Geometry check sheet. Reference: the model listing, model coordinates, mm. Face numbers are marked on the shaded views. A direction names the side the tool comes from. Round coordinates to 2 decimals unless told otherwise and drop trailing zeros. Write each loop counter-clockwise with the first axis right and the second up, starting at its lowest first coordinate (ties: lowest second). Pieces come first, ordered by that corner, then holes. Notation, with made-up numbers: M 68.25,69 L 91.25,69 A30 ccw 91.25,101 Z; hole C 55,23.25 d2. An arc over 180 degrees is marked long. Use a Markdown table: item, result.
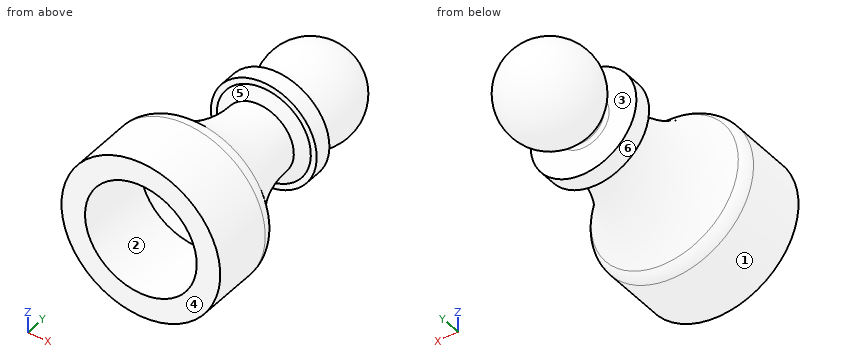
```python
from build123d import *

# Parameters (mm, degrees)
CHAMFER1_SIZE = 2
FILLET1_R     = 3
FILLET2_R     = 0.5


with BuildPart() as part:
    # Sketch1 → Revolve1 (revolve)
    with BuildSketch(Plane.XY, mode=Mode.PRIVATE) as revolve1_sk:
        with BuildLine():
            Line((9.5, 13.045692134), (9.5, 0))
            Line((9.5, 0), (13.5, 0))
            Line((13.5, 0), (13.5, 12))
            ThreePointArc((13.5, 12), (7.655959241, 19.576158489), (6, 29))
            Line((6, 29), (9, 29))
            Line((9, 29), (9, 32))
            Line((9, 32), (3.872983346, 32))
            Line((3.872983346, 32), (3.872983346, 33))
            ThreePointArc((3.872983346, 33), (7.745966692, 42), (0, 48))
            Line((0, 48), (0, 40))
            Line((0, 40), (0, 37))
            Line((0, 37), (0, 34.783882181))
            Line((0, 34.783882181), (0, 32))
            Line((0, 32), (3.954315273, 27.64896262))
            ThreePointArc((3.954315273, 27.64896262), (5.387413027, 19.838550851), (9.5, 13.045692134))
        make_face()
    revolve(revolve1_sk.sketch.rotate(Axis((0, 37, 0), (0, 1, 0)), 90), axis=Axis((0, 37, 0), (0, 1, 0)))

    # Chamfer1
    # the kernel refuses this chamfer: 2, 1.204425644 mm, written as the material it adds along each edge
    with BuildSketch(Plane(origin=(0, 29, 0), x_dir=(0, 0, -1), z_dir=(1, 0, 0))) as chamfer1_piece_1:
        with BuildLine():
            Line((5.955041017, -1.180657619), (6 + CHAMFER1_SIZE, 0))
            Line((6 + CHAMFER1_SIZE, 0), (6, 0))
            ThreePointArc((6, 0), (5.968001768, -0.611258692), (5.955041017, -1.180657619))
        make_face()
    revolve(axis=Axis((0, 29, 0), (0, 1, 0)))

    # Fillet1
    fillet1_edges = [part.edges().sort_by_distance(p)[0] for p in [
        (0, 12, 13.5),
    ]]
    fillet(fillet1_edges, radius=FILLET1_R)

    # Fillet2
    fillet2_edges = [part.edges().sort_by_distance(p)[0] for p in [
        (0, 33, 3.872983346),
        (0, 32, 3.872983346),
    ]]
    fillet(fillet2_edges, radius=FILLET2_R)


solid = part.part
```
Item 1: Cross-section at B-B, the plane y = 44.5. Record the cut outline in (x, z), and give its area (3 significant figures).
Outcome:
| item | result |
|---|---|
| outline | C 0,0 d13.23 |
| area | 137 mm2 |
Item 2: Mould release check, pull along X, two halves, no side actions. Record for the marked faces 1, 2 and 3: +X half, -X half, draft (parallel to the pull), parting line (faces both ways), or undercut.
Outcome:
| item | result |
|---|---|
| face 1 | parting line |
| face 2 | undercut |
| face 3 | draft |
Item 3: Go/stop test with flat-tipped pins: pin 1 (12 mm diameter, centred on y = 29.5, z = 5, fed in from -X); pin 2 (3 mm diameter, centred on x = 1, y = 21, fed in from -Z); pin 3 (5 mm diameter, centred on x = -10.5, y = 9.5, fed in from +Z). Record where each tip stops, or that it passes through.
Outcome:
| item | result |
|---|---|
| pin 1 | stops at x = -9 |
| pin 2 | stops at z = -7.64 |
| pin 3 | stops at z = 10.87 |
Item 4: Material ranges on line 1 along Y through (x, z) = (1.25, -7.25); line 2 along X through (y, z) = (7.5, 0); line 3 along X through (y, z) = (23, -4), recorded low to high. Write a range as from..to.
Outcome:
| item | result |
|---|---|
| line 1 | y = 15.9..20.29, 28.63..32, 36.86..43.14 |
| line 2 | x = -13.5..-9.5, 9.5..13.5 |
| line 3 | x = -5.13..-1.95, 1.95..5.13 |
Item 5: Access from +Z, -Z, +X, -X, +Y, -Y to the whole of each face (thin tool, end or side, straight path). Record for the marked faces 4, 5 and 6.
Outcome:
| item | result |
|---|---|
| face 4 | +Z, -Z, +X, -X, -Y |
| face 5 | none |
| face 6 | +Y |
Item 6: Cross-section at A-A, the plane y = 19. Record the cut outline in (x, z).
Outcome:
| item | result |
|---|---|
| outline | C 0,0 d15.84; hole C 0,0 d11.45 |
